Input: part model. Units: mm. Frame: model coordinates. A direction names the side the tool comes from. Coordinates: 2 decimals unless noted, no trailing zeros. Write each loop counter-clockwise with the first axis right and the second up, starting at its lowest first coordinate (ties: lowest second). Pieces come first, ordered by that corner, then holes. Notation, with made-up numbers: (83, 75) - (141, 75) arc R20 cw to (141, 99) - close; hole circle Ø11 at (9.5, 77). An arc over 180 degrees is marked (long way). Use CSV: the item, a comma, the result in double quotes.
```python
from build123d import *

# Parameters (mm, degrees)
SKETCH_1_W          = 40
SKETCH_1_H          = 40
EXTRUDE_1_DEPTH     = 5
SKETCH_2_R          = 4.05
CUT_EXTRUDE_1_DEPTH = 5
EXTRUDE_2_DEPTH     = 600
EXTRUDE_START       = 5
SKETCH_4_W          = 40
SKETCH_4_H          = 40
SKETCH_4_R          = 4.05
EXTRUDE_3_DEPTH     = 5
SKETCH_5_R          = 4.05
CUT_EXTRUDE_2_DEPTH = 5
SKETCH_6_R          = 4.05
CUT_EXTRUDE_3_DEPTH = 5


with BuildPart() as part:
    # 草图1 → 凸台-拉伸1 (new body)
    with BuildSketch(Plane(origin=(0, 0, 0), x_dir=(1, 0, 0), z_dir=(0, 1, 0))):
        Rectangle(SKETCH_1_W, SKETCH_1_H)
    extrude(amount=EXTRUDE_1_DEPTH)

    # 草图2 → 切除-拉伸1 (cut)
    with BuildSketch(Plane(origin=(0, 5, 0), x_dir=(1, 0, 0), z_dir=(0, 1, 0))):
        with Locations(Location((0, 0, 0), (0, 0, 270))):
            Circle(SKETCH_2_R)
    extrude(amount=-CUT_EXTRUDE_1_DEPTH, mode=Mode.SUBTRACT)

    # 草图3 → 凸台-拉伸2 (add)
    with BuildSketch(Plane(origin=(0, 5, 0), x_dir=(1, 0, 0), z_dir=(0, 1, 0))):
        Polygon((-20, 20), (-20, -20), (-15, -20), (-15, 15), (20, 15), (20, 20), align=None)
    extrude_2 = extrude(amount=EXTRUDE_2_DEPTH)

    # 镜向1: 凸台-拉伸2 across plane
    add(extrude_2.mirror(Plane.ZX.offset(605)))

    # 草图4 → 凸台-拉伸3 (add)
    with BuildSketch(Plane(origin=(0, 1205, 0), x_dir=(1, 0, 0), z_dir=(0, 1, 0)).offset(EXTRUDE_START)):
        Rectangle(SKETCH_4_W, SKETCH_4_H)
        with Locations(Location((0, 0, 0), (0, 0, 270))):
            Circle(SKETCH_4_R, mode=Mode.SUBTRACT)
    extrude(amount=-EXTRUDE_3_DEPTH)

    # 草图5 → 切除-拉伸2 (cut)
    with BuildSketch(Plane.XY.offset(-15)):
        with Locations((0, 20)):
            Circle(SKETCH_5_R)
    cut_extrude_2 = extrude(amount=-CUT_EXTRUDE_2_DEPTH, mode=Mode.SUBTRACT)

    # 镜向2: 切除-拉伸2 across plane
    add(cut_extrude_2.mirror(Plane(origin=(0, 605, 0), x_dir=(0, 0, 1), z_dir=(0, -1, 0))), mode=Mode.SUBTRACT)

    # 草图6 → 切除-拉伸3 (cut)
    with BuildSketch(Plane(origin=(-15, 0, 0), x_dir=(0, 0, -1), z_dir=(1, 0, 0))):
        with Locations((0, 20)):
            Circle(SKETCH_6_R)
    cut_extrude_3 = extrude(amount=-CUT_EXTRUDE_3_DEPTH, mode=Mode.SUBTRACT)

    # 镜向3: 切除-拉伸3 across plane
    add(cut_extrude_3.mirror(Plane(origin=(0, 605, 0), x_dir=(0, 0, 1), z_dir=(0, -1, 0))), mode=Mode.SUBTRACT)


solid = part.part
```
(1) Cut plane A-A on z = 11.5. Return loops of the section in (x, y), and give its area (3 significant figures).
Check values:
outline,"(-20, 0) - (20, 0) - (20, 5) - (-15, 5) - (-15, 1205) - (20, 1205) - (20, 1210) - (-20, 1210) - close"
area,"6,400 mm^2"
(2) Cut plane B-B on y = 755. Return loops of the section in (x, z), and give its area (3 significant figures).
Check values:
outline,"(-20, -20) - (20, -20) - (20, -15) - (-15, -15) - (-15, 20) - (-20, 20) - close"
area,"375 mm^2"
(3) Draft query along Y for faces 3 (the flat face through (4.2, 0, -0.3)), 4 (the flat face through (2, 5, 6)), 5 (the flat face through (2, 1205, 6)), 6 (the flat face through (20, 608, -18)). Return one class per face: pulls with the +Y half, pulls with the -Y half, needs draft (parallel to the pull), parting line crosses it, or undercut.
Check values:
face 3,"pulls with the -Y half"
face 4,"undercut"
face 5,"undercut"
face 6,"needs draft"
(4) Ray query, probe 1 along Y at (x, z) = (-18, 0); probe 2 along Y at (x, z) = (0.5, -6.5); probe 3 along Z at (x, y) = (-17, 1190). Return the intervals inside material, ascending. Write a range as from..to.
Check values:
probe 1,"0..15.95, 24.05..1185.95, 1194.05..1210"
probe 2,"0..5, 1205..1210"
probe 3,"-20..-4.05, 4.05..20"
(5) Reachability of faces 1 (the flat face through (-15, 613, 3)), 2 (the flat face through (0, 613, -20)) from +Z, -Z, +X, -X, +Y, -Y: full face, straight path, thin tool, end or side. Return the list, or none.
Check values:
face 1,"+Z, +X"
face 2,"-Z, +X, -X, +Y, -Y"
(6) Pin query (flat end, axial travel): pin 1 Ø10 at (y, z) = (492.5, 11) entering from +X; pin 2 Ø6 at (x, y) = (5.5, 463) entering from +Z. Return the tip coordinate at first contact, or that it passes through.
Check values:
pin 1,"x = -15"
pin 2,"z = -15"
